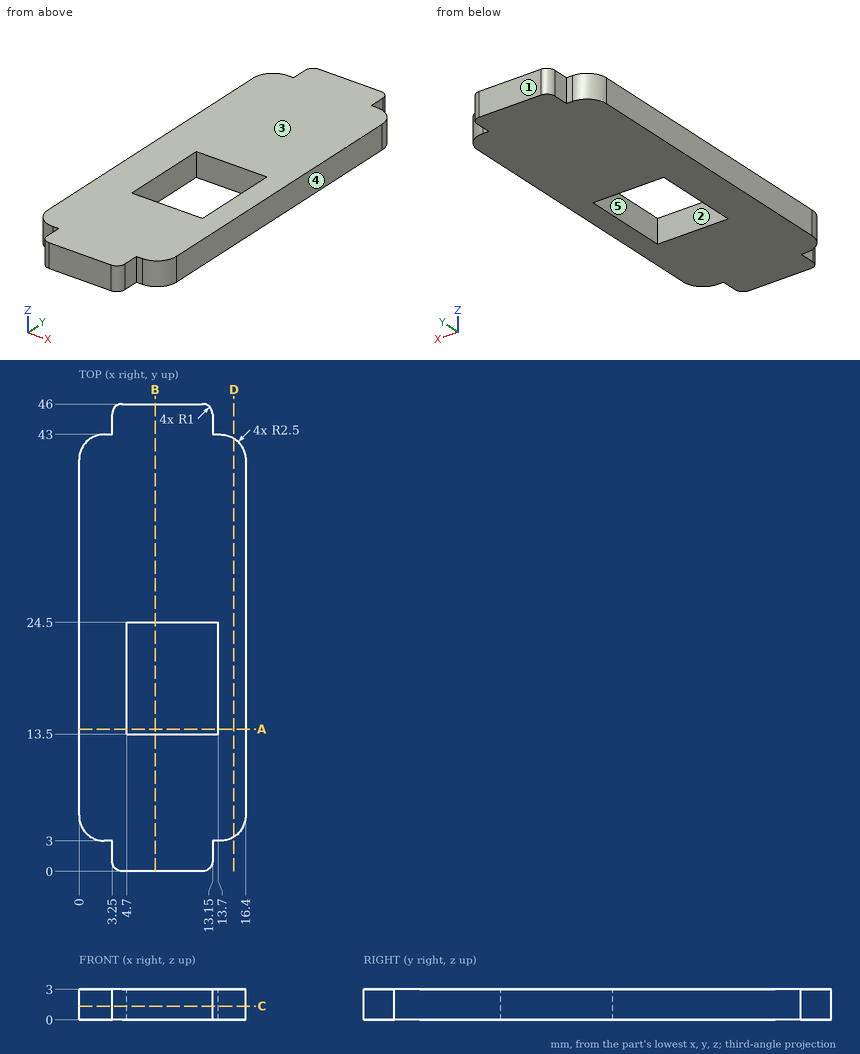
Input: dimensioned drawing with shaded views. Units: mm. Origin: part minimum x, y, z. A direction names the side the tool comes from. Coordinates: 2 decimals unless noted, no trailing zeros. Order: outer loops, then holes, each group sorted by start corner. A loop starts at its lowest first (then second) coordinate and runs counter-clockwise, first axis right, second up. Notation, with made-up numbers: (54.25, 74.25) - (64.25, 74.25) arc R14 cw to (64.25, 85.25) - close; hole circle Ø4 at (45, -8.75). An arc over 180 degrees is marked (long way). Return JSON: item names as keys, results as strings. Group by question number.
1. Cut plane B-B (x = 7.5). Output: boundary loops of the cut face in (y, z), plus the area to 3 significant figures.
2. Cut plane D-D (x = 15.25). Output: boundary loops of the cut face in (y, z), plus the area to 3 significant figures.
3. Cut plane A-A (y = 14). Output: boundary loops of the cut face in (x, z), plus the area to 3 significant figures.
4. Pin query (flat end, axial travel): pin 1 (1 mm diameter, centred on y = 44, z = 1, fed in from -X); pin 2 (1 mm diameter, centred on y = 1.5, z = 1, fed in from +X). Return the tip coordinate at first contact, or that it passes through.
5. Cut plane C-C (z = 1.35). Output: boundary loops of the cut face in (x, y), plus the area to 3 significant figures.
6. Material intervals for line 1 along X through (y, z) = (22, 2); line 2 along Y through (x, z) = (10.75, 0.6); line 3 along Y through (x, z) = (2.5, 1.2), sorted ascending. Write a range as [from, to].
7. Set-up query: the marked faces 1 and 2. Return all of +Z, -Z, +X, -X, +Y, -Y with unobstructed straight access to the full face (end or side cutting, diameter ignored); none if empty.
8. Pull-direction query (X, two-part tool) for the marked faces 3, 4 and 5; classes: pulls with the +X half, pulls with the -X half, needs draft (parallel to the pull), parting line crosses it, or undercut.
Resolved:
{
 "1": {"outline": "(0, 0) - (13.5, 0) - (13.5, 3) - (0, 3) - close; (24.5, 0) - (46, 0) - (46, 3) - (24.5, 3) - close", "area": "105 mm²"},
 "2": {"outline": "(3.4, 0) - (42.6, 0) - (42.6, 3) - (3.4, 3) - close", "area": "118 mm²"},
 "3": {"outline": "(0, 0) - (4.7, 0) - (4.7, 3) - (0, 3) - close; (13.7, 0) - (16.4, 0) - (16.4, 3) - (13.7, 3) - close", "area": "22.2 mm²"},
 "4": {"pin 1": "stops at x = 3.25", "pin 2": "stops at x = 13.15"},
 "5": {"outline": "(0, 5.5) arc R2.5 ccw to (2.5, 3) - (3.25, 3) - (3.25, 1) arc R1 ccw to (4.25, 0) - (12.15, 0) arc R1 ccw to (13.15, 1) - (13.15, 3) - (13.9, 3) arc R2.5 ccw to (16.4, 5.5) - (16.4, 40.5) arc R2.5 ccw to (13.9, 43) - (13.15, 43) - (13.15, 45) arc R1 ccw to (12.15, 46) - (4.25, 46) arc R1 ccw to (3.25, 45) - (3.25, 43) - (2.5, 43) arc R2.5 ccw to (0, 40.5) - close; hole (4.7, 13.5) - (13.7, 13.5) - (13.7, 24.5) - (4.7, 24.5) - close", "area": "610 mm²"},
 "6": {"line 1": "x = [0, 4.7], [13.7, 16.4]", "line 2": "y = [0, 13.5], [24.5, 46]", "line 3": "y = [3, 43]"},
 "7": {"face 1": "+Z, -Z, +X, -X, +Y", "face 2": "+Z, -Z"},
 "8": {"face 3": "needs draft", "face 4": "pulls with the +X half", "face 5": "undercut"}
}
